Autodesk Inventor part; units mm, degrees
ref_plane "YZ Plane" through (0, 0, 0) normal (1, 0, 0) x (0, 1, 0)
ref_plane "XZ Plane" through (0, 0, 0) normal (0, 1, 0) x (-1, 0, 0)
ref_plane "XY Plane" through (0, 0, 0) normal (0, 0, 1) x (1, 0, 0)
sketch "Sketch15" plane through (0, 0, 0) normal (0, 0, 1) x (1, 0, 0)
  line L0 (0, 0) -> (0, 2.5)
  line L1 (0, 2.5) -> (2, 2.5)
  line L2 (3, 4.4) -> (3, 4.4)
  line L3 (2, 1.5) -> (11, 1.5)
  line L4 (11, 0) -> (0, 0)
  line L5 (11, 0) -> (7.2, 0)
  line L6 (2, 1.5) -> (2, 2.5)
  line L7 (11, 1.5) -> (11, 0)
  dimension "d84" = 1.5
  dimension "d87" = 2.5
  dimension "d116" = 2
  dimension "d117" = 9
revolve "Revolution1" add sketch "Sketch15" angle 360 about axis through (11, 0, 0) along (-1, 0, 0)
chamfer "Chamfer5" distance 0.2 angle 45 1 edges at (11, -1.5, 0)
thread "Thread8"
sketch "Sketch20" plane through (0, 0, 0) normal (-1, 0, 0) x (0, 0, 1)
  line L0 (-1.25, 0.7217) -> (0, 1.4434)
  line L1 (0, 1.4434) -> (1.25, 0.7217)
  line L2 (1.25, 0.7217) -> (1.25, -0.7217)
  line L3 (1.25, -0.7217) -> (0, -1.4434)
  line L4 (0, -1.4434) -> (-1.25, -0.7217)
  line L5 (-1.25, -0.7217) -> (-1.25, 0.7217)
  point P0 (0, 0)
  point P1 (0, 0)
  dimension "d143" = 2.5
extrude "Extrusion19" cut sketch "Sketch20" against normal blind 1.5
chamfer "Chamfer6" distance 0.2 angle 45 1 edges at (0, -2.5, 0)
properties part number "Bolt3RH"
Check sheet for the modelled part. Datum: model origin and axes. Units: mm. A direction names the side the tool comes from. Give positions to 0.01 mm unless a question says otherwise; leave off trailing zeros. Loops run counter-clockwise (first coordinate to the right, second up) from the corner with the lowest first, then second, coordinate; pieces in that order, holes last. Notation, with made-up numbers: M 19.25,28 L 76.25,28 A20 cw 76.25,46 Z; hole C 5,19.25 d8. An arc over 180 degrees is marked long. Answer as CSV lines item,"result".
Item 1: Depth check by flat-ended pin: pin 1 Ø1.5 at (x, z) = (1.5, -1) entering from +Y; pin 2 Ø1 at (x, y) = (4.5, -0.5) entering from +Z; pin 3 Ø2 at (y, z) = (-0.5, 0.5) entering from -X; pin 4 Ø1.5 at (x, z) = (3.5, -1) entering from -Y. Enter the tip coordinate at first touch or a pass-through.
Reply:
pin 1,"y = 2.49"
pin 2,"z = 1.5"
pin 3,"x = 0"
pin 4,"y = -1.48"
Item 2: Sectioned sample at B-B, the plane x = 5. Enter the section's corners in (y, z).
Reply:
outline,"C 0,0 d3"
Item 3: Set-up check for faces 4 (the face through (1, 0, -1.25)), 5 (the face through (11, 0, 0)), 6 (the face through (6.46, -1.5, 0.07)): record each of +Z, -Z, +X, -X, +Y, -Y from which the full face is reachable in a straight line by a thin tool's end or side.
Reply:
face 4,"-X"
face 5,"+Z, -Z, +X, +Y, -Y"
face 6,"+X"
Item 4: Sectioned sample at A-A, the plane y = 0. Enter the section's corners in (x, z), then the cut area to 3 significant figures.
Reply:
outline,"M 0,-2.3 L 0.2,-2.5 L 2,-2.5 L 2,-1.5 L 10.8,-1.5 L 11,-1.3 L 11,1.3 L 10.8,1.5 L 2,1.5 L 2,2.5 L 0.2,2.5 L 0,2.3 L 0,1.25 L 1.5,1.25 L 1.5,-1.25 L 0,-1.25 Z"
area,"33.2 mm^2"
Item 5: Draft check along Z on faces 1 (the face through (1.5, 0, 0)), 2 (the face through (0, 0, 2)), 3 (the face through (1.11, -0.54, -2.44)). Enter one of: pulls with the +Z half, pulls with the -Z half, needs draft (parallel to the pull), parting line crosses it, or undercut.
Reply:
face 1,"undercut"
face 2,"needs draft"
face 3,"parting line crosses it"
Item 6: Scan lines: L1, parallel to X at y = -0.3, z = -0.45; L2, parallel to X at y = 1.55, z = -1.4; L3, parallel to Z at x = 7, y = -0.4. Record each from-to range of solid material in increasing order.
Reply:
L1,"1.5 to 11"
L2,"0 to 2"
L3,"-1.45 to 1.45"
